Can you work these out from the model? Positions are in its coordinate system, mm. A direction names the side the tool comes from. Round coordinates to 2 decimals unless told otherwise and drop trailing zeros.
```python
from build123d import *

# Parameters (mm, degrees)
SKETCH1_W                                       = 15.875
SKETCH1_H                                       = 15.875
BOSS_EXTRUDE1_DEPTH                             = 497.84
SKETCH8_R                                       = 6.8199
CUT_EXTRUDE1_DEPTH                              = 13.08608
L_0_29_DIAMETER_HOLE1_D                         = 7.366
L_0_29_DIAMETER_HOLE1_DEPTH                     = 50.8
L_0_29_DIAMETER_HOLE1_TIP                       = 2.21296966
CBORE_FOR_10_SOCKET_HEAD_CAP_SCREW1_D           = 4.9784
CBORE_FOR_10_SOCKET_HEAD_CAP_SCREW1_DEPTH       = 25.4
CBORE_FOR_10_SOCKET_HEAD_CAP_SCREW1_CBORE_D     = 9.525
CBORE_FOR_10_SOCKET_HEAD_CAP_SCREW1_CBORE_DEPTH = 4.826
CBORE_FOR_10_SOCKET_HEAD_CAP_SCREW1_TIP         = 1.495662253
CBORE_FOR_10_SOCKET_HEAD_CAP_SCREW2_D           = 4.9784
CBORE_FOR_10_SOCKET_HEAD_CAP_SCREW2_DEPTH       = 25.4
CBORE_FOR_10_SOCKET_HEAD_CAP_SCREW2_CBORE_D     = 9.525
CBORE_FOR_10_SOCKET_HEAD_CAP_SCREW2_CBORE_DEPTH = 4.826
CBORE_FOR_10_SOCKET_HEAD_CAP_SCREW2_TIP         = 1.495662253


with BuildPart() as part:
    # Sketch1 → Boss-Extrude1 (new body)
    with BuildSketch(Plane.XY):
        with Locations((7.9375, 7.9375)):
            Rectangle(SKETCH1_W, SKETCH1_H)
    extrude(amount=BOSS_EXTRUDE1_DEPTH)

    # Sketch8 → Cut-Extrude1 (cut)
    with BuildSketch(Plane.ZY):
        with Locations((465.6201, 7.9375)):
            Circle(SKETCH8_R)
        with Locations((32.2199, 7.9375)):
            Circle(SKETCH8_R)
    extrude(amount=-CUT_EXTRUDE1_DEPTH, mode=Mode.SUBTRACT)

    # L (0.29) Diameter Hole1
    with Locations(Plane.ZY.offset(-13.08608)):
        with Locations((32.2199, 7.9375), (465.6201, 7.9375)):
            Hole(L_0_29_DIAMETER_HOLE1_D / 2, depth=L_0_29_DIAMETER_HOLE1_DEPTH)
            with Locations((0, 0, -(L_0_29_DIAMETER_HOLE1_DEPTH + L_0_29_DIAMETER_HOLE1_TIP / 2))):  # 118° drill point
                Cone(0, L_0_29_DIAMETER_HOLE1_D / 2, L_0_29_DIAMETER_HOLE1_TIP, mode=Mode.SUBTRACT)

    # CBORE for #10 Socket Head Cap Screw1
    with Locations(Plane(origin=(-863.724136144, 0, -1707.973131805), x_dir=(-1, 0, 0), z_dir=(0, -1, 0))):
        with Locations((-404.936636144, -2199.813131805), (-404.936636144, -2186.413131805), (-871.661636144, -2186.413131805), (-871.661636144, -2199.813131805)):
            CounterBoreHole(CBORE_FOR_10_SOCKET_HEAD_CAP_SCREW1_D / 2, CBORE_FOR_10_SOCKET_HEAD_CAP_SCREW1_CBORE_D / 2, CBORE_FOR_10_SOCKET_HEAD_CAP_SCREW1_CBORE_DEPTH, depth=CBORE_FOR_10_SOCKET_HEAD_CAP_SCREW1_DEPTH)
            with Locations((0, 0, -(CBORE_FOR_10_SOCKET_HEAD_CAP_SCREW1_DEPTH + CBORE_FOR_10_SOCKET_HEAD_CAP_SCREW1_TIP / 2))):  # 118° drill point
                Cone(0, CBORE_FOR_10_SOCKET_HEAD_CAP_SCREW1_D / 2, CBORE_FOR_10_SOCKET_HEAD_CAP_SCREW1_TIP, mode=Mode.SUBTRACT)

    # CBORE for #10 Socket Head Cap Screw2
    with Locations(Plane(origin=(-863.724136144, 0, -1707.973131805), x_dir=(-1, 0, 0), z_dir=(0, -1, 0))):
        with Locations((-404.936636144, -1713.973131805), (-404.936636144, -1727.373131805), (-871.661636144, -1713.973131805), (-871.661636144, -1727.373131805)):
            CounterBoreHole(CBORE_FOR_10_SOCKET_HEAD_CAP_SCREW2_D / 2, CBORE_FOR_10_SOCKET_HEAD_CAP_SCREW2_CBORE_D / 2, CBORE_FOR_10_SOCKET_HEAD_CAP_SCREW2_CBORE_DEPTH, depth=CBORE_FOR_10_SOCKET_HEAD_CAP_SCREW2_DEPTH)
            with Locations((0, 0, -(CBORE_FOR_10_SOCKET_HEAD_CAP_SCREW2_DEPTH + CBORE_FOR_10_SOCKET_HEAD_CAP_SCREW2_TIP / 2))):  # 118° drill point
                Cone(0, CBORE_FOR_10_SOCKET_HEAD_CAP_SCREW2_D / 2, CBORE_FOR_10_SOCKET_HEAD_CAP_SCREW2_TIP, mode=Mode.SUBTRACT)


solid = part.part
```
(1) We'd pull the mould along Z, two halves only. Please class faces 1 (the cylindrical face through (8.97, 2.38, 483.09)), 2 (the flat face through (8, 8, 0)), 3 (the flat face through (8, 0, 245)): released by +Z, released by -Z, zero draft, split by the parting line, or undercut.
(2) If I drill on line 1 (X direction, y = 12.5, z = 19.4) (3 decimals); line 2 (Z direction, x = 2.5, y = 12.5); line 3 (Z direction, x = 5.25, y = 6.75), over which ranges is the centre line in solid material (lowest first)?
(3) For pin 1 (5.5 mm diameter, centred on x = 7.94, z = 19.4, fed in from -Y), with a flat end and sliding along its axis, tell me the tip position at first contact or that it passes through.
(4) Which directions (+Z, -Z, +X, -X, +Y, -Y) give clear straight access to the entire face, cutting with the end or side of a thin tool? Please do faces 4 (the cylindrical face through (6.451, 8.237, 25.407)), 5 (the flat face through (6, 4.826, 494)), 6 (the flat face through (15.875, 8, 245)).
Check result:
1. face 1: undercut
1. face 2: released by -Z
1. face 3: zero draft
2. line 1: x = 0 to 5.448, 10.427 to 15.875
2. line 2: z = 0 to 27.15, 37.29 to 460.55, 470.69 to 497.84
2. line 3: z = 0 to 25.5, 38.94 to 458.9, 472.34 to 497.84
3. pin 1: stops at y = 4.83
4. face 4: -X
4. face 5: -Y
4. face 6: +Z, -Z, +X, +Y, -Y
